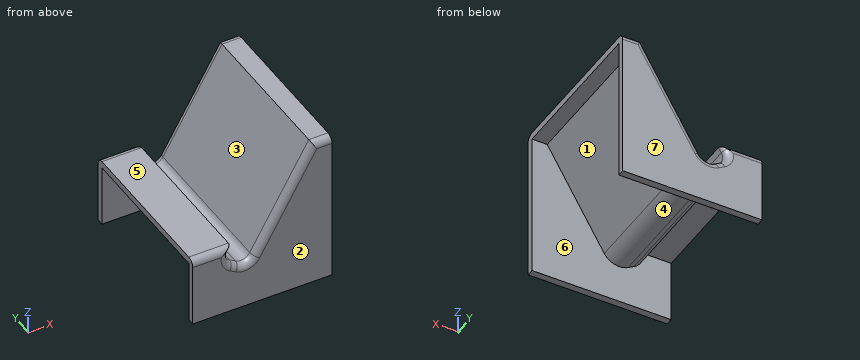
```python
from build123d import *

# Parameters (mm, degrees)
F0_W         = 60
F0_H         = 30
F1_DEPTH     = 60
F2_R         = 7.5
F3_T1_DEPTH  = 38.8119784648
F3_T3_DEPTH  = 97.3760430703
F3_T5_DEPTH  = 5
F3_T7_DEPTH  = 16.5470053838
F3_T9_DEPTH  = 53.4529946162
F3_T12_ANGLE = 90
F3_T14_ANGLE = 90
F3_T16_ANGLE = 90
F3_T18_ANGLE = 90
F4_T         = 5


# Not quite as in the source:
# - a fillet or chamfer that OpenCascade refuses, or shapes differently, is made with other operations: its cross-section is extruded or revolved along the edge and cut away or added
# - a shell that OpenCascade refuses in one call is made with other operations: the cavity is built on its own and cut out


with BuildPart() as f1:
    # F0 (on Front) → F1 (new body, symmetric)
    with BuildSketch(Plane.XZ):
        Polygon((46.1880215352, 80), (0, 0), (60, 0), (60, 80), align=None)
        with Locations((30, -15)):
            Rectangle(F0_W, F0_H)
        Polygon((0, -30), (0, 0), (-17.3205080757, 10), (-11.5470053838, 20), (-40, 20), (-40, -30), align=None)
    extrude(amount=F1_DEPTH, both=True)

    # F2
    f2_edges = [f1.edges().sort_by_distance(p)[0] for p in [
        (-17.320508, 0, 10),
        (0, 0, 0),
    ]]
    fillet(f2_edges, radius=F2_R)

    # F3: fillet of radius 5 on 14 edges, made by hand

    # F3_s2 → F3_t1 (cut)
    with BuildSketch(Plane.YZ.offset(33.6880215352)):
        with BuildLine():
            ThreePointArc((-55, 80), (-58.5355339059, 78.5355339059), (-60, 75))
            Line((-60, 75), (-60, 80))
            Line((-60, 80), (-55, 80))
        make_face()
        with BuildLine():
            ThreePointArc((60, 75), (58.5355339059, 78.5355339059), (55, 80))
            Line((55, 80), (60, 80))
            Line((60, 80), (60, 75))
        make_face()
    extrude(amount=F3_T1_DEPTH, mode=Mode.SUBTRACT)

    # F3_s4 → F3_t3 (cut)
    with BuildSketch(Plane(origin=(52.4380215352, 0, 90.8253175473), x_dir=(0, 1, 0), z_dir=(-0.5, 0, -0.8660254038))):
        with BuildLine():
            ThreePointArc((-55, 0), (-58.5355339059, 1.4644660941), (-60, 5))
            Line((-60, 5), (-60, 0))
            Line((-60, 0), (-55, 0))
        make_face()
        with BuildLine():
            ThreePointArc((55, 0), (58.5355339059, 1.4644660941), (60, 5))
            Line((60, 5), (60, 0))
            Line((60, 0), (55, 0))
        make_face()
    extrude(amount=F3_T3_DEPTH, mode=Mode.SUBTRACT)

    # F3_s6 → F3_t5 (cut)
    with BuildSketch(Plane(origin=(-6.4951905284, 0, 3.75), x_dir=(0, 1, 0), z_dir=(-0.8660254038, 0, 0.5))):
        with BuildLine():
            ThreePointArc((-60, 5), (-58.5355339059, 1.4644660941), (-55, 0))
            Line((-55, 0), (-60, 0))
            Line((-60, 0), (-60, 5))
        make_face()
        with BuildLine():
            ThreePointArc((60, 5), (58.5355339059, 1.4644660941), (55, 0))
            Line((55, 0), (60, 0))
            Line((60, 0), (60, 5))
        make_face()
    extrude(amount=F3_T5_DEPTH, mode=Mode.SUBTRACT)

    # F3_s8 → F3_t7 (cut)
    with BuildSketch(Plane(origin=(3.75, 0, 6.4951905284), x_dir=(0, 1, 0), z_dir=(0.5, 0, 0.8660254038))):
        with BuildLine():
            ThreePointArc((-60, 25), (-58.5355339059, 21.4644660941), (-55, 20))
            Line((-55, 20), (-60, 20))
            Line((-60, 20), (-60, 25))
        make_face()
        with BuildLine():
            ThreePointArc((60, 25), (58.5355339059, 21.4644660941), (55, 20))
            Line((55, 20), (60, 20))
            Line((60, 20), (60, 25))
        make_face()
    extrude(amount=F3_T7_DEPTH, mode=Mode.SUBTRACT)

    # F3_s10 → F3_t9 (cut)
    with BuildSketch(Plane.YZ.offset(-52.5)):
        with BuildLine():
            ThreePointArc((-60, 15), (-58.5355339059, 18.5355339059), (-55, 20))
            Line((-55, 20), (-60, 20))
            Line((-60, 20), (-60, 15))
        make_face()
        with BuildLine():
            ThreePointArc((60, 15), (58.5355339059, 18.5355339059), (55, 20))
            Line((55, 20), (60, 20))
            Line((60, 20), (60, 15))
        make_face()
    extrude(amount=F3_T9_DEPTH, mode=Mode.SUBTRACT)

    # F3_s11 → F3_t12 (revolve, cut)
    with BuildSketch(Plane(origin=(3.75, 0, 6.4951905284), x_dir=(0, 1, 0), z_dir=(0.5, 0, 0.8660254038))):
        with BuildLine():
            ThreePointArc((60, -5), (58.5355339059, -1.4644660941), (55, 0))
            Line((55, 0), (60, 0))
            Line((60, 0), (60, -5))
        make_face()
    revolve(axis=Axis((-2.7451905284, 60, 10.2451905284), (0, 1, 0)), revolution_arc=F3_T12_ANGLE, mode=Mode.SUBTRACT)

    # F3_s13 → F3_t14 (revolve, cut)
    with BuildSketch(Plane(origin=(3.75, 0, 6.4951905284), x_dir=(0, 1, 0), z_dir=(0.5, 0, 0.8660254038))):
        with BuildLine():
            ThreePointArc((60, 25), (58.5355339059, 21.4644660941), (55, 20))
            Line((55, 20), (60, 20))
            Line((60, 20), (60, 25))
        make_face()
    revolve(axis=Axis((-7.0753175473, 60, 12.7451905284), (0, -1, 0)), revolution_arc=F3_T14_ANGLE, mode=Mode.SUBTRACT)

    # F3_s15 → F3_t16 (revolve, cut)
    with BuildSketch(Plane(origin=(3.75, 0, 6.4951905284), x_dir=(0, 1, 0), z_dir=(0.5, 0, 0.8660254038))):
        with BuildLine():
            ThreePointArc((-55, 0), (-58.5355339059, -1.4644660941), (-60, -5))
            Line((-60, -5), (-60, 0))
            Line((-60, 0), (-55, 0))
        make_face()
    revolve(axis=Axis((-2.7451905284, -60, 10.2451905284), (0, 1, 0)), revolution_arc=F3_T16_ANGLE, mode=Mode.SUBTRACT)

    # F3_s17 → F3_t18 (revolve, cut)
    with BuildSketch(Plane(origin=(3.75, 0, 6.4951905284), x_dir=(0, 1, 0), z_dir=(0.5, 0, 0.8660254038))):
        with BuildLine():
            ThreePointArc((-60, 25), (-58.5355339059, 21.4644660941), (-55, 20))
            Line((-55, 20), (-60, 20))
            Line((-60, 20), (-60, 25))
        make_face()
    revolve(axis=Axis((-7.0753175473, -60, 12.7451905284), (0, -1, 0)), revolution_arc=F3_T18_ANGLE, mode=Mode.SUBTRACT)

    # F4: shell of thickness 5, made by hand


with BuildPart() as f4_core1:
    # F4_t2: copy of F1
    add(f1.part)

    # the walls: a layer under each face that stays
    f4_faces = [f4_core1.faces().sort_by_distance(p)[0] for p in [
        (24.9690107676, 0, 43.2475952642),
        (53.0940107676, 0, 80),
        (-0.8040476901, 0, 3.0007468312),
        (-23.3333333333, -60, -12.5),
        (-8.6602540378, 0, 5),
        (-23.3333333333, 60, -12.5),
        (-14.3197612445, 0, 10.8040476901),
        (-25.7735026919, 0, 20),
        (-12.5587567297, 0, 18.2475952642),
    ]]
    thicken(f4_faces, amount=-F4_T, mode=Mode.SUBTRACT)


with BuildPart() as f1_1:
    add(f1.part)

    # what is left inside the walls is the cavity
    f4_cavity = [f4_core1.part.solids().sort_by_distance(p)[0] for p in [
        (59.95, 18.333333, 22.5),
    ]]
    add(f4_cavity, mode=Mode.SUBTRACT)


solid = f1_1.part
```
Work out the finished part from the listing and answer in its coordinate system (mm). Face numbers are marked on the shaded views. A direction names the side the tool comes from. Coordinates: 2 decimals unless noted, no trailing zeros. Write each loop counter-clockwise with the first axis right and the second up, starting at its lowest first coordinate (ties: lowest second). Pieces come first, ordered by that corner, then holes. Notation, with made-up numbers: (27, 26) - (36, 26) arc R22 ccw to (36, 40) - close; hole circle Ø3 at (48, -31.75). An arc over 180 degrees is marked (long way). Answer as a JSON object with one key per item and string values.
Q1. Find section A-A (z = -17). Write down the section's boundary in (x, y).
Results list:
{"outline": "(-40, -60) - (60, -60) - (60, -55) - (-40, -55) - close; (-40, 55) - (60, 55) - (60, 60) - (-40, 60) - close"}
Q2. Find section B-B (x = -25). Write down the section's boundary in (y, z), plus the area to 3 significant figures.
Results list:
{"outline": "(-60, -30) - (-55, -30) - (-55, 15) - (55, 15) - (55, -30) - (60, -30) - (60, 15) arc R5 ccw to (55, 20) - (-55, 20) arc R5 ccw to (-60, 15) - close", "area": "1,040 mm^2"}
Q3. Consider L1, parallel to Y at x = 47.5, z = 29; L2, parallel to Z at x = -26, y = -14; L3, parallel to X at y = 23, z = 17. Determine where each line is inside the solid, lowest interval first. Write a range as from..to.
Results list:
{"L1": "y = -60..-55, 55..60", "L2": "z = 15..20", "L3": "x = -40..-13.28, 9.81..15.59"}
Q4. For a pull along Y with two mould halves and no side action, classify the marked faces 5, 6 and 7 as pulls with the +Y half, pulls with the -Y half, needs draft (parallel to the pull), parting line crosses it, or undercut.
Results list:
{"face 5": "needs draft", "face 6": "undercut", "face 7": "pulls with the +Y half"}
Q5. Given pin 1 Ø10 at (y, z) = (7, -9) entering from -X; pin 2 Ø8 at (y, z) = (-7, -4.5) entering from -X; pin 3 Ø5 at (y, z) = (-13, 47) entering from -X; pin 4 Ø5.5 at (x, y) = (55, -22.5) entering from -Z, each flat-ended and moving along its own axis, determine where each tip first touches the part or whether it passes through.
Results list:
{"pin 1": "passes through", "pin 2": "stops at x = -9.13", "pin 3": "stops at x = 25.69", "pin 4": "stops at z = 75"}
Q6. Find section C-C (y = -17). Write down the section's boundary in (x, z).
Results list:
{"outline": "(-40, 15) - (-19.37, 15) arc R12.5 ccw to (-13.33, 1.92) - (-9, -0.58) arc R12.5 ccw to (8.08, 4) - (49.07, 75) - (60, 75) - (60, 80) - (46.19, 80) - (3.75, 6.5) arc R7.5 cw to (-6.5, 3.75) - (-10.83, 6.25) arc R7.5 cw to (-13.57, 16.5) - (-11.55, 20) - (-40, 20) - close"}
Q7. Which of the six approach directions +Z, -Z, +X, -X, +Y, -Y give full straight-line access (tool end or side, diameter ignored) to the marked faces 1, 2, 3 and 4?
Results list:
{"face 1": "-Z, +X", "face 2": "+Z, -Z, +X, -X, -Y", "face 3": "+Z, +Y, -Y", "face 4": "-Z"}
